```python
from build123d import *

# Parameters (mm, degrees)
CYLINDER004_R     = 1.9
CYLINDER004_DEPTH = 20
CYLINDER005_R     = 4
CYLINDER005_DEPTH = 13


with BuildPart() as cylinder004:
    # Cylinder004 → Cylinder004 (new body)
    with BuildSketch(Plane.XY.offset(-1)):
        Circle(CYLINDER004_R)
    extrude(amount=CYLINDER004_DEPTH)


with BuildPart() as cut004:
    # Cylinder005 → Cylinder005 (new body)
    with BuildSketch(Plane.XY):
        Circle(CYLINDER005_R)
    extrude(amount=CYLINDER005_DEPTH)

    # Cut004: cut Cylinder004
    add(cylinder004.part, mode=Mode.SUBTRACT)


solid = cut004.part
```
Here's how the part is built. I have some questions about the finished solid (model axes, mm). Coordinates: 2 decimals unless noted, no trailing zeros. Order: outer loops, then holes, each group sorted by start corner. A loop starts at its lowest first (then second) coordinate and runs counter-clockwise, first axis right, second up.
Item 1: If we section it at D-D, the plane x = 3.5: List the corners of the cut face in (y, z) for me, then the cut area to 3 significant figures.
Response values:
outline: (-1.94, 0) - (1.94, 0) - (1.94, 13) - (-1.94, 13) - close
area: 50.3 mm2
Item 2: If we section it at C-C, the plane z = 2.5: List the corners of the cut face in (x, y) for me, then the cut area to 3 significant figures.
Response values:
outline: circle Ø8 at (0, 0); hole circle Ø3.8 at (0, 0)
area: 38.9 mm2
Item 3: Thinking about a two-plate mould opening in X: for faces 1 (the face through (2, -1, 0)), 2 (the face through (-0.867, -3.905, 6.409)), 3 (the face through (-1.9, 0.08, 6.41)), which applies, pulls with the +X half, pulls with the -X half, needs draft (parallel to the pull), parting line crosses it, or undercut?
Response values:
face 1: needs draft
face 2: parting line crosses it
face 3: undercut
Item 4: I need wall thicknesses on probe 1 along Y at (x, z) = (0, 2.75); probe 2 along X at (y, z) = (0.75, 4); probe 3 along Y at (x, z) = (-0.5, 5.5). Which ranges of each line are inside material? Lowest first, please.
Response values:
probe 1: y = -4 to -1.9, 1.9 to 4
probe 2: x = -3.93 to -1.75, 1.75 to 3.93
probe 3: y = -3.97 to -1.83, 1.83 to 3.97
Item 5: If we section it at A-A, the plane y = 0: List the corners of the cut face in (x, z) for me, then the cut area to 3 significant figures.
Response values:
outline: (-4, 0) - (-1.9, 0) - (-1.9, 13) - (-4, 13) - close; (1.9, 0) - (4, 0) - (4, 13) - (1.9, 13) - close
area: 54.6 mm2
Item 6: I'm going to push flat-ended pins straight in: pin 1 Ø4.5 at (x, y) = (0, 0) entering from +Z; pin 2 Ø1.5 at (x, z) = (-1.5, 11) entering from +Y; pin 3 Ø1 at (x, z) = (-2.5, 11.5) entering from +Y; pin 4 Ø4 at (y, z) = (-2.5, 6) entering from +X. Where does each tip first touch, or does it pass through?
Response values:
pin 1: stops at z = 13
pin 2: stops at y = 3.93
pin 3: stops at y = 3.46
pin 4: stops at x = 3.97
